Autodesk Inventor part; units mm, degrees
ref_plane "YZ Plane" through (0, 0, 0) normal (1, 0, 0) x (0, 1, 0)
ref_plane "XZ Plane" through (0, 0, 0) normal (0, 1, 0) x (-1, 0, 0)
ref_plane "XY Plane" through (0, 0, 0) normal (0, 0, 1) x (1, 0, 0)
sketch "Sketch1" plane through (0, 0, 0) normal (0, 0, 1) x (1, 0, 0)
  line L0 (0, 69) -> (3, 69)
  line L1 (3, 69) -> (3, 78)
  line L2 (3, 0) -> (3, 9)
  line L3 (3, 9) -> (0, 9)
  line L4 (0, 49) -> (3, 49)
  line L5 (3, 29) -> (0, 29)
  line L6 (15, 41.5) -> (15, 36.5)
  line L7 (12, 41.5) -> (12, 43)
  line L8 (12, 43) -> (7, 43)
  line L9 (7, 43) -> (7, 41.5)
  line L10 (12, 36.5) -> (12, 35)
  line L11 (12, 35) -> (7, 35)
  line L12 (7, 35) -> (7, 36.5)
  line L13 (0, 69) -> (0, 49)
  line L14 (0, 29) -> (0, 9)
  line L15 (3, 49) -> (3, 41.5)
  line L16 (3, 36.5) -> (3, 29)
  line L17 (15, 36.5) -> (12, 36.5)
  line L18 (7, 36.5) -> (3, 36.5)
  line L19 (3, 41.5) -> (7, 41.5)
  line L20 (12, 41.5) -> (15, 41.5)
  line L21 (57, 69) -> (54, 69)
  line L22 (54, 69) -> (54, 78)
  line L23 (54, 0) -> (54, 9)
  line L24 (54, 9) -> (57, 9)
  line L25 (57, 49) -> (54, 49)
  line L26 (54, 29) -> (57, 29)
  line L27 (42, 41.5) -> (42, 36.5)
  line L28 (45, 41.5) -> (45, 43)
  line L29 (45, 43) -> (50, 43)
  line L30 (50, 43) -> (50, 41.5)
  line L31 (45, 36.5) -> (45, 35)
  line L32 (45, 35) -> (50, 35)
  line L33 (50, 35) -> (50, 36.5)
  line L34 (57, 69) -> (57, 49)
  line L35 (57, 29) -> (57, 9)
  line L36 (54, 49) -> (54, 41.5)
  line L37 (54, 36.5) -> (54, 29)
  line L38 (42, 36.5) -> (45, 36.5)
  line L39 (50, 36.5) -> (54, 36.5)
  line L40 (54, 41.5) -> (50, 41.5)
  line L41 (45, 41.5) -> (42, 41.5)
  line L42 (3, 0) -> (54, 0)
  line L43 (54, 78) -> (3, 78)
  line L44 (24.2574, 22.636) -> (34.864, 33.2426)
  line L45 (34.864, 33.2426) -> (32.7426, 35.364)
  line L46 (32.7426, 35.364) -> (22.136, 24.7574)
  line L47 (22.136, 24.7574) -> (24.2574, 22.636)
  line L48 (20.0147, 26.8787) -> (30.6213, 37.4853)
  line L49 (30.6213, 37.4853) -> (28.5, 39.6066)
  line L50 (28.5, 39.6066) -> (17.8934, 29)
  line L51 (17.8934, 29) -> (20.0147, 26.8787)
  line L52 (28.5, 18.3934) -> (39.1066, 29)
  line L53 (39.1066, 29) -> (36.9853, 31.1213)
  line L54 (36.9853, 31.1213) -> (26.3787, 20.5147)
  line L55 (26.3787, 20.5147) -> (28.5, 18.3934)
  line L56 (24.2574, 22.636) -> (34.864, 33.2426)
  line L57 (34.864, 33.2426) -> (32.7426, 35.364)
  line L58 (32.7426, 35.364) -> (22.136, 24.7574)
  line L59 (22.136, 24.7574) -> (24.2574, 22.636)
  circle A0 centre (19, 40.5) radius 1
  circle A1 centre (38, 40.5) radius 1
  point P0 (0, 0)
  point P1 (57, 56.3821)
  point P2 (13.5, 36.5)
  point P3 (43.5, 41.5)
  dimension "d58" = 3
  dimension "d59" = 4
  dimension "d60" = 5
  dimension "d61" = 3
  dimension "d62" = 3
  dimension "d63" = 4
  dimension "d64" = 5
  dimension "d65" = 3
  dimension "d66" = 3
  dimension "d77" = 6
  dimension "d80" = 6
  dimension "d83" = 2
  dimension "d84" = 2
  dimension "d85" = 4
  dimension "d86" = 4
  dimension "d87" = 4
  dimension "d88" = 4
extrude "Extrusion1" add sketch "Sketch1" along normal blind 3
properties part number "Motor_Mount_Front"
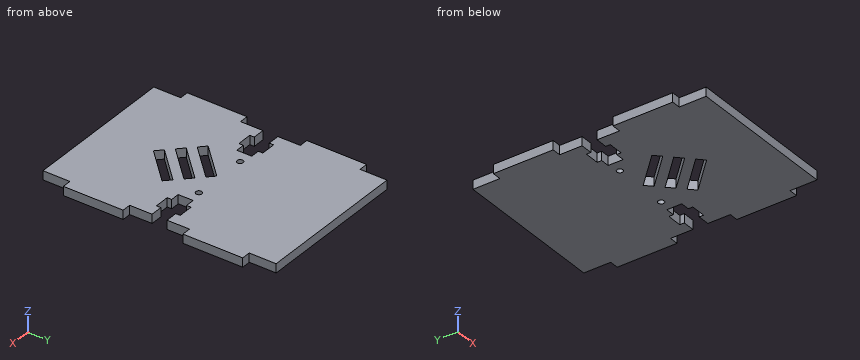
The listing builds one solid part. Answer for the finished solid, in the listing's coordinates (mm). Coordinates: 2 decimals unless noted, no trailing zeros. Write each loop counter-clockwise with the first axis right and the second up, starting at its lowest first coordinate (ties: lowest second). Pieces come first, ordered by that corner, then holes. Notation, with made-up numbers: (43, 50.5) - (68, 50.5) arc R9 ccw to (68, 55.5) - close; hole circle Ø11 at (6.25, -25.75). An arc over 180 degrees is marked (long way). Put each result on its own line as item: value.
1. The part is cut by section C-C on x = 31.5. Give the vertices of the cut face in (y, z).
Answer sheet:
outline: (0, 0) - (21.39, 0) - (21.39, 3) - (0, 3) - close; (25.64, 0) - (29.88, 0) - (29.88, 3) - (25.64, 3) - close; (34.12, 0) - (78, 0) - (78, 3) - (34.12, 3) - close
2. The part is cut by section D-D on z = 0.95. State how many separate pieces and enclosed holes the cut face has, plus the area to 3 significant figures.
Answer sheet:
separate pieces: 1
enclosed holes: 5
area: 3,930 mm^2
3. Find the intervals of material crossed by line 1 along Y through (x, z) = (10, 2.8); line 2 along X through (y, z) = (41, 1.1); line 3 along Y through (x, z) = (24, 1.6), in increasing order. Write a range as from..to.
Answer sheet:
line 1: y = 0..35, 43..78
line 2: x = 15..18.13, 19.87..37.13, 38.87..42
line 3: y = 0..22.89, 26.62..30.86, 35.11..78
4. The part is cut by section B-B on y = 40.5. Give the vertices of the cut face in (x, z), plus the area to 3 significant figures.
Answer sheet:
outline: (15, 0) - (18, 0) - (18, 3) - (15, 3) - close; (20, 0) - (37, 0) - (37, 3) - (20, 3) - close; (39, 0) - (42, 0) - (42, 3) - (39, 3) - close
area: 69.0 mm^2
5. The part is cut by section A-A on x = 53. Give the vertices of the cut face in (y, z), plus the area to 3 significant figures.
Answer sheet:
outline: (0, 0) - (36.5, 0) - (36.5, 3) - (0, 3) - close; (41.5, 0) - (78, 0) - (78, 3) - (41.5, 3) - close
area: 219 mm^2
6. Flat-ended cylindrical pins translate along their axes: pin 1 Ø1.5 at (x, z) = (1.5, 1) entering from +Y; pin 2 Ø0.9 at (y, z) = (6, 1) entering from +X; pin 3 Ø0.9 at (y, z) = (38, 1) entering from +X. Find the tip coordinate at first contact, or state that the pin passes through.
Answer sheet:
pin 1: stops at y = 69
pin 2: stops at x = 54
pin 3: stops at x = 42
